Verification items for the finished model (mm, model axes). A direction names the side the tool comes from. Coordinates: 2 decimals unless noted, no trailing zeros. Order: outer loops, then holes, each group sorted by start corner. A loop starts at its lowest first (then second) coordinate and runs counter-clockwise, first axis right, second up. Notation, with made-up numbers: M 64,-40 L 112,-40 A26 ccw 112,-9 Z; hole C -12,-17.75 d3. An arc over 180 degrees is marked long. Use one line per item in the form item = value. Start each with the question number.
```python
from build123d import *

# Parameters (mm, degrees)
F0_W      = 100
F0_H      = 60
F1_DEPTH  = 30
F2_T      = -3
F3_W      = 9
F3_H      = 9
F3_W_2    = 3
F3_H_2    = 3
F4_DEPTH  = 27
F5_R      = 1.65
F6_DEPTH  = 100.001
F7_R      = 1.65
F8_DEPTH  = 5
F9_R      = 1.65
F10_DEPTH = 5
F12_DEPTH = 1


with BuildPart() as f1:
    # F0 (on Top) → F1 (new body)
    with BuildSketch(Plane.XY):
        Rectangle(F0_W, F0_H)
    extrude(amount=F1_DEPTH)

    # F2
    f2_openings = [f1.faces().sort_by_distance(p)[0] for p in [
        (0, 0, 30),
    ]]
    offset(amount=F2_T, openings=f2_openings)

    # F3 (on face) → F4 (join)
    with BuildSketch(Plane.XY.offset(3)):
        with Locations((-42.5, 22.5)):
            Rectangle(F3_W, F3_H)
        with Locations((42.5, 22.5)):
            Rectangle(F3_W, F3_H)
        with Locations((45.5, -25.5)):
            Rectangle(F3_W_2, F3_H_2)
        with Locations((-45.5, -25.5)):
            Rectangle(F3_W_2, F3_H_2)
    extrude(amount=F4_DEPTH)

    # F5 (on face) → F6 (cut, through all)
    with BuildSketch(Plane.YZ.offset(50)):
        with Locations((25, 25)):
            Circle(F5_R)
    extrude(amount=-F6_DEPTH, mode=Mode.SUBTRACT)

    # F7 (on face) → F8 (cut)
    with BuildSketch(Plane.YZ.offset(50)):
        with BuildLine():
            ThreePointArc((25, 21), (27.8284271247, 22.1715728753), (29, 25))
            ThreePointArc((29, 25), (25, 29), (21, 25))
            ThreePointArc((21, 25), (22.1715728753, 22.1715728753), (25, 21))
        make_face()
        with Locations((25, 25)):
            Circle(F7_R, mode=Mode.SUBTRACT)
        with BuildLine():
            ThreePointArc((21, 25), (25, 29), (29, 25))
            ThreePointArc((29, 25), (27.8284271247, 22.1715728753), (25, 21))
            Line((25, 21), (30, 21))
            Line((30, 21), (30, 30))
            Line((30, 30), (21, 30))
            Line((21, 30), (21, 25))
        make_face()
    extrude(amount=-F8_DEPTH, mode=Mode.SUBTRACT)

    # F9 (on face) → F10 (cut)
    with BuildSketch(Plane(origin=(-50, 0, 0), x_dir=(0, -1, 0), z_dir=(-1, 0, 0))):
        with BuildLine():
            ThreePointArc((-25, 21), (-22.1715728753, 22.1715728753), (-21, 25))
            ThreePointArc((-21, 25), (-27.8284271247, 27.8284271247), (-25, 21))
        make_face()
        with Locations((-25, 25)):
            Circle(F9_R, mode=Mode.SUBTRACT)
        with BuildLine():
            ThreePointArc((-25, 21), (-27.8284271247, 27.8284271247), (-21, 25))
            Line((-21, 25), (-21, 30))
            Line((-21, 30), (-30, 30))
            Line((-30, 30), (-30, 21))
            Line((-30, 21), (-25, 21))
        make_face()
    extrude(amount=-F10_DEPTH, mode=Mode.SUBTRACT)

    # F11 (on face) → F12 (cut)
    with BuildSketch(Plane.XZ.offset(30)):
        with BuildLine():
            ThreePointArc((-3, 30), (0, 27), (3, 30))
            Line((3, 30), (-3, 30))
        make_face()
    extrude(amount=-F12_DEPTH, mode=Mode.SUBTRACT)


solid = f1.part
```
1. Material ranges on line 1 along Y through (x, z) = (-40.75, 25); line 2 along Y through (x, z) = (-29.5, 27); line 3 along Z through (x, y) = (-40, 25), recorded low to high.
2. Cross-section at A-A on y = 0. Enter the section's corners in (x, z), and give its area (3 significant figures).
3. Release check for a two-part mould opening along Y. For faces 4 (the flat face through (-4, -29, 30)), 5 (the flat face through (-48, 21, 27)), 6 (the flat face through (38, 22, 16)) record: pulls with the +Y half, pulls with the -Y half, needs draft (parallel to the pull), parting line crosses it, or undercut.
4. Tool access check on faces 1 (the flat face through (-44, -26, 16)), 2 (the cylindrical face through (-47.535, 22.203, 22.141)), 3 (the cylindrical face through (47.535, 22.141, 22.203)). Record the directions out of +Z, -Z, +X, -X, +Y, -Y that give a thin tool (end or side, any length) a straight path to the whole face; none if there is none.
5. Depth check by flat-ended pin: P1, Ø1.5, axis at x = -47.5, y = 28, coming from the +Z side; P2, Ø2.5, axis at y = 27.5, z = 26, coming from the -X side; P3, Ø2.5, axis at y = 25, z = 25, coming from the +X side; P4, Ø2.5, axis at x = 0.5, z = 28.5, coming from the -Y side. Enter the tip coordinate at first touch or a pass-through.
6. Cross-section at C-C on x = 35. Enter the section's corners in (y, z).
7. Cross-section at D-D on x = 0. Enter the section's corners in (y, z), and give its area (3 significant figures).
8. Cross-section at B-B on z = 19. Enter the section's corners in (x, y).
Final values:
q1.line_1 = -30 to -27, 18 to 23.35, 26.65 to 30
q1.line_2 = -30 to -27, 27 to 30
q1.line_3 = 0 to 23.35, 26.65 to 30
q2.outline = M -50,0 L 50,0 L 50,30 L 47,30 L 47,3 L -47,3 L -47,30 L -50,30 Z
q2.area = 462 mm2
q3.face_4 = needs draft
q3.face_5 = pulls with the +Y half
q3.face_6 = undercut
q4.face_1 = +Z
q4.face_2 = +Z, -X, +Y
q4.face_3 = +Z, +X, +Y
q5.P1 = 21
q5.P2 = -45
q5.P3 = through
q5.P4 = -29
q6.outline = M -30,0 L 30,0 L 30,30 L 27,30 L 27,3 L -27,3 L -27,30 L -30,30 Z
q7.outline = M -30,0 L 30,0 L 30,30 L 27,30 L 27,3 L -27,3 L -27,30 L -29,30 L -29,27 L -30,27 Z
q7.area = 339 mm2
q8.outline = M -50,-30 L 50,-30 L 50,30 L -50,30 Z; hole M -47,-24 L -44,-24 L -44,-27 L 44,-27 L 44,-24 L 47,-24 L 47,18 L 38,18 L 38,27 L -38,27 L -38,18 L -47,18 Z
